The model under review builds one solid part; all positions refer to its coordinate system, in mm. A direction names the side the tool comes from. Coordinates: 2 decimals unless noted, no trailing zeros. Order: outer loops, then holes, each group sorted by start corner. A loop starts at its lowest first (then second) coordinate and runs counter-clockwise, first axis right, second up. Notation, with made-up numbers: M -14.5,66.5 L 40.5,66.5 A28 cw 40.5,95.5 Z; hole C -21.5,-7.75 d8. An arc over 180 degrees is marked long. One line per item, written item: value.
```python
from build123d import *

# Parameters (mm, degrees)
BOSS_EXTRUDE1_DEPTH = 18


with BuildPart() as part:
    # Sketch1 → Boss-Extrude1 (new body)
    with BuildSketch(Plane.XY):
        with BuildLine():
            Line((4.070181983, 148.487708827), (4.070181983, 43.487708827))
            Line((4.070181983, 43.487708827), (104.070181983, -56.512291173))
            Line((104.070181983, -56.512291173), (104.070181983, -166.512291173))
            Line((104.070181983, -166.512291173), (-95.929818017, -166.512291173))
            Line((-95.929818017, -166.512291173), (-95.929818017, -36.512291173))
            Line((-95.929818017, -36.512291173), (-125.929818017, -6.512291173))
            Line((-125.929818017, -6.512291173), (-125.929818017, 148.487708827))
            ThreePointArc((-125.929818017, 148.487708827), (-124.465351923, 152.023242733), (-120.929818017, 153.487708827))
            Line((-120.929818017, 153.487708827), (-95.929818017, 153.487708827))
            Line((-95.929818017, 153.487708827), (-0.929818017, 153.487708827))
            ThreePointArc((-0.929818017, 153.487708827), (2.605715889, 152.023242733), (4.070181983, 148.487708827))
        make_face()
    extrude(amount=BOSS_EXTRUDE1_DEPTH)


solid = part.part
```
(1) We need section A-A, the plane z = 5. State the section outline as (x, y) points.
Geometry results:
outline: M -125.93,-6.51 L -95.93,-36.51 L -95.93,-166.51 L 104.07,-166.51 L 104.07,-56.51 L 4.07,43.49 L 4.07,148.49 A5 ccw -0.93,153.49 L -120.93,153.49 A5 ccw -125.93,148.49 Z
(2) Insertion check: pin 1 Ø6 at (y, z) = (75, 7.5) entering from +X; pin 2 Ø5 at (x, y) = (21, 33) entering from -Z; pin 3 Ø4 at (x, z) = (15, 11.5) entering from +Y. Each pin has a flat end and moves straight along its axis. Give the tip position at first contact, or say it passes through.
Geometry results:
pin 1: stops at x = 4.07
pin 2: passes through
pin 3: stops at y = 34.56
(3) Tool access review of faces 1 (the flat face through (4.07, 97, 9)), 2 (the flat face through (-95.93, -102, 9)), 3 (the flat face through (-35, -4, 18)): name each direction out of +Z, -Z, +X, -X, +Y, -Y from which nothing blocks a thin tool from reaching the whole face with its end or side.
Geometry results:
face 1: +Z, -Z, +X, +Y
face 2: +Z, -Z, -X, -Y
face 3: +Z, +X, -X, +Y, -Y
(4) We need section C-C, the plane x = 59. State the section outline as (y, z) points, plus the area to 3 significant figures.
Geometry results:
outline: M -166.51,0 L -11.44,0 L -11.44,18 L -166.51,18 Z
area: 2,790 mm2
(5) We need section B-B, the plane y = -65. State the section outline as (x, z) points.
Geometry results:
outline: M -95.93,0 L 104.07,0 L 104.07,18 L -95.93,18 Z
(6) For L1, parallel to X at y = 114, z = 14.5; L2, parallel to X at y = -135.5, z = 13.25; L3, parallel to Y at x = 87.5, z = 1.5, list the stretches that pass through material, from the lowest coordinate up.
Geometry results:
L1: x = -125.93 to 4.07
L2: x = -95.93 to 104.07
L3: y = -166.51 to -39.94
